Source: three-view drawing plus pictorial views. Frame: mm from the lowest corner of the part. Give positions to 0.01 mm unless a question says otherwise; leave off trailing zeros. Order: outer loops, then holes, each group sorted by start corner. A loop starts at its lowest first (then second) coordinate and runs counter-clockwise, first axis right, second up. Notation, with made-up numbers: (22, -28.75) - (61, -28.75) arc R25 cw to (61, -16.75) - close; hole circle Ø4 at (5.5, 0.5). An arc over 180 degrees is marked (long way). Answer in a Markdown table with one row per item. Add a question column.
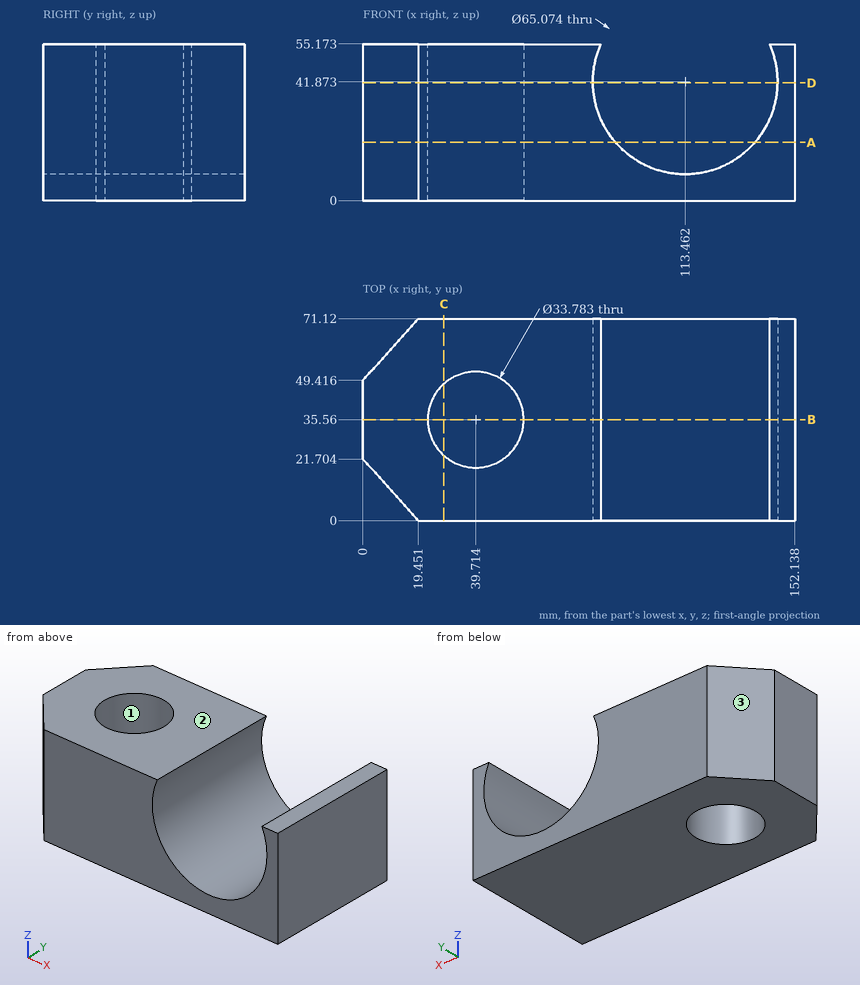
Q1. Pull-direction query (Y, two-part tool) for the marked faces 1, 2 and 3; classes: +Y half, -Y half, draft (parallel to the pull), parting line (faces both ways), or undercut.
Q2. Section D-D, the plane z = 41.5. Return loops of the section in (x, y) (1 decimal), then the cut area to 3 significant figures.
Q3. Section A-A, the plane z = 20.5. Return loops of the section in (x, y) (1 decimal), then the cut area to 3 significant figures.
Q4. Line query: probe 1 along X at (y, z) = (35, 41); probe 2 along X at (y, z) = (25, 31.5) (1 decimal); probe 3 along X at (y, z) = (53.5, 21.5) (1 decimal). Output: solid intervals per line, ascending.
Q5. Section C-C, the plane x = 28.5. Return loops of the section in (y, z), then the cut area to 3 significant figures.
Q6. Section B-B, the plane y = 35.56. Return loops of the section in (x, z), then the cut area to 3 significant figures.
Computed:
| question | item | result |
|---|---|---|
| 1 | face 1 | undercut |
| 1 | face 2 | draft |
| 1 | face 3 | +Y half |
| 2 | outline | (0, 21.7) - (19.5, 0) - (80.9, 0) - (80.9, 71.1) - (19.5, 71.1) - (0, 49.4) - close; (146, 0) - (152.1, 0) - (152.1, 71.1) - (146, 71.1) - close; hole circle Ø33.8 at (39.7, 35.6) |
| 2 | area | 4,870 mm^2 |
| 3 | outline | (0, 21.7) - (19.5, 0) - (88.9, 0) - (88.9, 71.1) - (19.5, 71.1) - (0, 49.4) - close; (138, 0) - (152.1, 0) - (152.1, 71.1) - (138, 71.1) - close; hole circle Ø33.8 at (39.7, 35.6) |
| 3 | area | 6,010 mm^2 |
| 4 | probe 1 | x = 0 to 22.83, 56.6 to 80.94, 145.99 to 152.14 |
| 4 | probe 2 | x = 0 to 26.5, 52.9 to 82.6, 144.3 to 152.1 |
| 4 | probe 3 | x = 3.7 to 88.1, 138.8 to 152.1 |
| 5 | outline | (0, 0) - (22.93, 0) - (22.93, 55.17) - (0, 55.17) - close; (48.19, 0) - (71.12, 0) - (71.12, 55.17) - (48.19, 55.17) - close |
| 5 | area | 2,530 mm^2 |
| 6 | outline | (0, 0) - (22.82, 0) - (22.82, 55.17) - (0, 55.17) - close; (56.61, 0) - (152.14, 0) - (152.14, 55.17) - (143.16, 55.17) arc R32.54 cw (long way) to (83.77, 55.17) - (56.61, 55.17) - close |
| 6 | area | 4,030 mm^2 |
